from build123d import *

# Parameters (mm, degrees)
BASE_DEPTH         = 25
SKETCH2_R          = 1.55
CUT_EXTRUDE1_DEPTH = 2
SKETCH4_R          = 1.55
CUT_EXTRUDE3_DEPTH = 47.368092477
CHAMFER2_SIZE      = 6
FILLET1_R          = 2
FILLET2_R          = 4


with BuildPart() as part:
    # Sketch1 → Base (new body)
    with BuildSketch(Plane.XY):
        Polygon((0, 0), (30, 0), (30, 2), (2, 2), (2, 25), (0, 25), align=None)
    extrude(amount=BASE_DEPTH)

    # Sketch2 → Cut-Extrude1 (cut)
    with BuildSketch(Plane.ZY):
        with Locations(Location((19.5, 18, 0), (0, 0, 270))):
            Circle(SKETCH2_R)
        with Locations(Location((7.5, 18, 0), (0, 0, 270))):
            Circle(SKETCH2_R)
    extrude(amount=-CUT_EXTRUDE1_DEPTH, mode=Mode.SUBTRACT)

    # Sketch4 → Cut-Extrude3 (cut, through all)
    with BuildSketch(Plane.XZ):
        with Locations(Location((10, 10.5, 0), (0, 0, 270))):
            Circle(SKETCH4_R)
        with Locations(Location((25, 21.5, 0), (0, 0, 270))):
            Circle(SKETCH4_R)
    extrude(amount=-CUT_EXTRUDE3_DEPTH, mode=Mode.SUBTRACT)

    # Chamfer2
    chamfer2_edges = [part.edges().sort_by_distance(p)[0] for p in [
        (30, 1, 0),
    ]]
    chamfer(chamfer2_edges, length=CHAMFER2_SIZE)

    # Fillet1
    fillet1_edges = [part.edges().sort_by_distance(p)[0] for p in [
        (2, 2, 12.5),
    ]]
    fillet(fillet1_edges, radius=FILLET1_R)

    # Fillet2
    fillet2_edges = [part.edges().sort_by_distance(p)[0] for p in [
        (0, 0, 12.5),
    ]]
    fillet(fillet2_edges, radius=FILLET2_R)


solid = part.part
Check sheet for the modelled part. Datum: model origin and axes. Units: mm. A direction names the side the tool comes from. Round coordinates to 2 decimals unless told otherwise and drop trailing zeros. Loops run counter-clockwise (first coordinate to the right, second up) from the corner with the lowest first, then second, coordinate; pieces in that order, holes last. Notation, with made-up numbers: (13, 82.25) -> (61, 82.25) arc R19 cw to (61, 115.25) -> close; hole circle Ø9 at (-32.75, -26.5). An arc over 180 degrees is marked (long way). Put each result on its own line as item: value. Start each with the question number.
1. Scan lines: probe 1 along Y at (x, z) = (25.5, 10.5); probe 2 along Z at (x, y) = (24.75, 1.5). Record each from-to range of solid material in increasing order.
2. Section check C-C (y = 18). Enter the section's corners in (x, z), plus the area to 3 significant figures.
3. Section check B-B (z = 7.5). Enter the section's corners in (x, y).
4. Draft check along Y on faces 1 (the face through (0.986, 16.568, 6.906)), 2 (the face through (1.203, 1.141, 12.675)), 3 (the face through (2.6, 2.57, 12.68)). Enter one of: +Y half, -Y half, draft (parallel to the pull), parting line (faces both ways), or undercut.
5. Gauge pin test, flat ends, axial feed: pin 1 (2.5 mm diameter, centred on x = 25, z = 21.5, fed in from +Y) (3 decimals); pin 2 (4 mm diameter, centred on x = 16.5, z = 14.5, fed in from +Y); pin 3 (8 mm diameter, centred on y = 10, z = 4.5, fed in from +X). Record the tip position at first contact, or that the pin passes through.
6. Section check A-A (x = 25). Enter the section's corners in (y, z), plus the area to 3 significant figures.
7. Section check D-D (x = 10). Enter the section's corners in (y, z).
8. Access from +Z, -Z, +X, -X, +Y, -Y to the whole of each face (thin tool, end or side, straight path). Record for faces 4 (the face through (2, 14, 12)), 5 (the face through (9.06, 0.99, 11.73)).
Findings:
1. probe 1: y = 0 to 2
1. probe 2: z = 0.75 to 19.97, 23.03 to 25
2. outline: (0, 0) -> (2, 0) -> (2, 5.95) -> (0, 5.95) -> close; (0, 9.05) -> (2, 9.05) -> (2, 17.95) -> (0, 17.95) -> close; (0, 21.05) -> (2, 21.05) -> (2, 25) -> (0, 25) -> close
2. area: 37.6 mm^2
3. outline: (0, 4) arc R4 ccw to (4, 0) -> (30, 0) -> (30, 2) -> (4, 2) arc R2 cw to (2, 4) -> (2, 16.45) -> (0, 16.45) -> close; (0, 19.55) -> (2, 19.55) -> (2, 25) -> (0, 25) -> close
4. face 1: undercut
4. face 2: -Y half
4. face 3: +Y half
5. pin 1: passes through
5. pin 2: stops at y = 2
5. pin 3: stops at x = 2
6. outline: (0, 1) -> (2, 1) -> (2, 19.95) -> (0, 19.95) -> close; (0, 23.05) -> (2, 23.05) -> (2, 25) -> (0, 25) -> close
6. area: 41.8 mm^2
7. outline: (0, 0) -> (2, 0) -> (2, 8.95) -> (0, 8.95) -> close; (0, 12.05) -> (2, 12.05) -> (2, 25) -> (0, 25) -> close
8. face 4: +Z, -Z, +X, +Y
8. face 5: +Y, -Y
